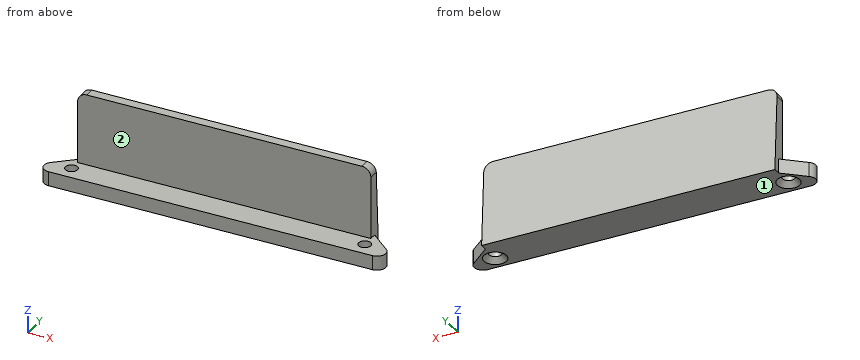
from build123d import *

# Parameters (mm, degrees)
BOSS_EXTRUDE1_DEPTH                             = 4
FILLET1_R                                       = 2.48
SKETCH4_W                                       = 81.9
SKETCH4_H                                       = 4
BOSS_EXTRUDE3_DEPTH                             = 2
SKETCH6_W                                       = 81.9
SKETCH6_H                                       = 4
BOSS_EXTRUDE4_DEPTH                             = 19.9
FILLET3_R                                       = 2.5
SKETCH7_W                                       = 81.9
SKETCH7_H                                       = 35.801674527
CUT_REVOLVE2_ANGLE                              = 3
CSK_FOR_M3_FLAT_HEAD_MACHINE_SCREW1_D           = 3.4
CSK_FOR_M3_FLAT_HEAD_MACHINE_SCREW1_DEPTH       = 10.1
CSK_FOR_M3_FLAT_HEAD_MACHINE_SCREW1_CSINK_D     = 6.3
CSK_FOR_M3_FLAT_HEAD_MACHINE_SCREW1_CSINK_ANGLE = 90
CSK_FOR_M3_FLAT_HEAD_MACHINE_SCREW1_TIP         = 1.021463052


with BuildPart() as part:
    # Sketch1 → Boss-Extrude1 (new body)
    with BuildSketch(Plane.XY):
        Polygon((-51.95, 0), (51.95, 0), (40.95, 9.408805716), (-40.95, 9.408805716), align=None)
    extrude(amount=BOSS_EXTRUDE1_DEPTH)

    # Fillet1
    fillet1_edges = [part.edges().sort_by_distance(p)[0] for p in [
        (51.95, 0, 2),
        (-51.95, 0, 2),
    ]]
    fillet(fillet1_edges, radius=FILLET1_R)

    # Sketch4 → Boss-Extrude3 (add)
    with BuildSketch(Plane(origin=(0, 9.408805716, 0), x_dir=(1, 0, 0), z_dir=(0, 1, 0))):
        with Locations((0, -2)):
            Rectangle(SKETCH4_W, SKETCH4_H)
    extrude(amount=BOSS_EXTRUDE3_DEPTH)

    # Sketch6 → Boss-Extrude4 (add)
    with BuildSketch(Plane.XY.offset(4)):
        with Locations((0, 9.408805716)):
            Rectangle(SKETCH6_W, SKETCH6_H)
    extrude(amount=BOSS_EXTRUDE4_DEPTH)

    # Fillet3
    fillet3_edges = [part.edges().sort_by_distance(p)[0] for p in [
        (-40.95, 9.408805716, 23.9),
        (40.95, 9.408805716, 23.9),
    ]]
    fillet(fillet3_edges, radius=FILLET3_R)

    # Sketch7 → Cut-Revolve2 (revolve, cut)
    with BuildSketch(Plane(origin=(0, 11.408805716, 0), x_dir=(1, 0, 0), z_dir=(0, 1, 0))):
        with Locations((0, -17.900837264)):
            Rectangle(SKETCH7_W, SKETCH7_H)
    revolve(axis=Axis((-40.95, 11.408805716, 0), (1, 0, 0)), revolution_arc=CUT_REVOLVE2_ANGLE, mode=Mode.SUBTRACT)

    # CSK for M3 Flat Head Machine Screw1
    with Locations(Plane(origin=(0, 0, 0), x_dir=(-1, 0, 0), z_dir=(0, 0, -1))):
        with Locations((-40.95, 4.158805716), (40.95, 4.158805716)):
            CounterSinkHole(CSK_FOR_M3_FLAT_HEAD_MACHINE_SCREW1_D / 2, CSK_FOR_M3_FLAT_HEAD_MACHINE_SCREW1_CSINK_D / 2, depth=CSK_FOR_M3_FLAT_HEAD_MACHINE_SCREW1_DEPTH, counter_sink_angle=CSK_FOR_M3_FLAT_HEAD_MACHINE_SCREW1_CSINK_ANGLE)
            with Locations((0, 0, -(CSK_FOR_M3_FLAT_HEAD_MACHINE_SCREW1_DEPTH + CSK_FOR_M3_FLAT_HEAD_MACHINE_SCREW1_TIP / 2))):  # 118° drill point
                Cone(0, CSK_FOR_M3_FLAT_HEAD_MACHINE_SCREW1_D / 2, CSK_FOR_M3_FLAT_HEAD_MACHINE_SCREW1_TIP, mode=Mode.SUBTRACT)


solid = part.part
Geometry: final body of the model. Coordinates: model frame, mm. Face numbers are marked on the shaded views. A direction names the side the tool comes from. Give positions to 0.01 mm unless a question says otherwise; leave off trailing zeros. Write each loop counter-clockwise with the first axis right and the second up, starting at its lowest first coordinate (ties: lowest second). Pieces come first, ordered by that corner, then holes. Notation, with made-up numbers: M -32.75,50.25 L 20.25,50.25 A24 ccw 20.25,60.25 Z; hole C 84.25,47.5 d7. An arc over 180 degrees is marked long. Answer in a Markdown table with one row per item. Add a question column.
(1) Section A-A on x = 13. Return loops of the section in (y, z), and give its area (3 significant figures).
(2) Section B-B on z = 9. Return loops of the section in (x, y).
(3) Reachability of the marked faces 1 and 2 from +Z, -Z, +X, -X, +Y, -Y: full face, straight path, thin tool, end or side. Return the list, or none.
(4) First-contact query: pin 1 (4.5 mm diameter, centred on x = -0.5, y = 3, fed in from +Z); pin 2 (6 mm diameter, centred on x = 20, z = 4.5, fed in from +Y); pin 3 (3 mm diameter, centred on x = 6, z = 10.5, fed in from -Y). Flat tips, straight axial feed; report the tip coordinate or a pass-through.
(5) Section C-C on z = 15.5. Return loops of the section in (x, y), and give its area (3 significant figures).
(6) Ray query, line 1 (Z direction, x = 14.5, y = 4.75); line 2 (X direction, y = 10.25, z = 6.5); line 3 (Y direction, x = -17, z = 4.75). Return the intervals inside material, ascending.
Result set:
| question | item | result |
|---|---|---|
| 1 | outline | M 0,0 L 11.41,0 L 10.16,23.9 L 7.41,23.9 L 7.41,4 L 0,4 Z |
| 1 | area | 110 mm^2 |
| 2 | outline | M -40.95,7.41 L 40.95,7.41 L 40.95,10.94 L -40.95,10.94 Z |
| 3 | face 1 | -Z, +X, -X, +Y, -Y |
| 3 | face 2 | +Z, +X, -X, -Y |
| 4 | pin 1 | stops at z = 4 |
| 4 | pin 2 | stops at y = 11.33 |
| 4 | pin 3 | stops at y = 7.41 |
| 5 | outline | M -40.95,7.41 L 40.95,7.41 L 40.95,10.6 L -40.95,10.6 Z |
| 5 | area | 261 mm^2 |
| 6 | line 1 | z = 0 to 4 |
| 6 | line 2 | x = -40.95 to 40.95 |
| 6 | line 3 | y = 7.41 to 11.16 |
